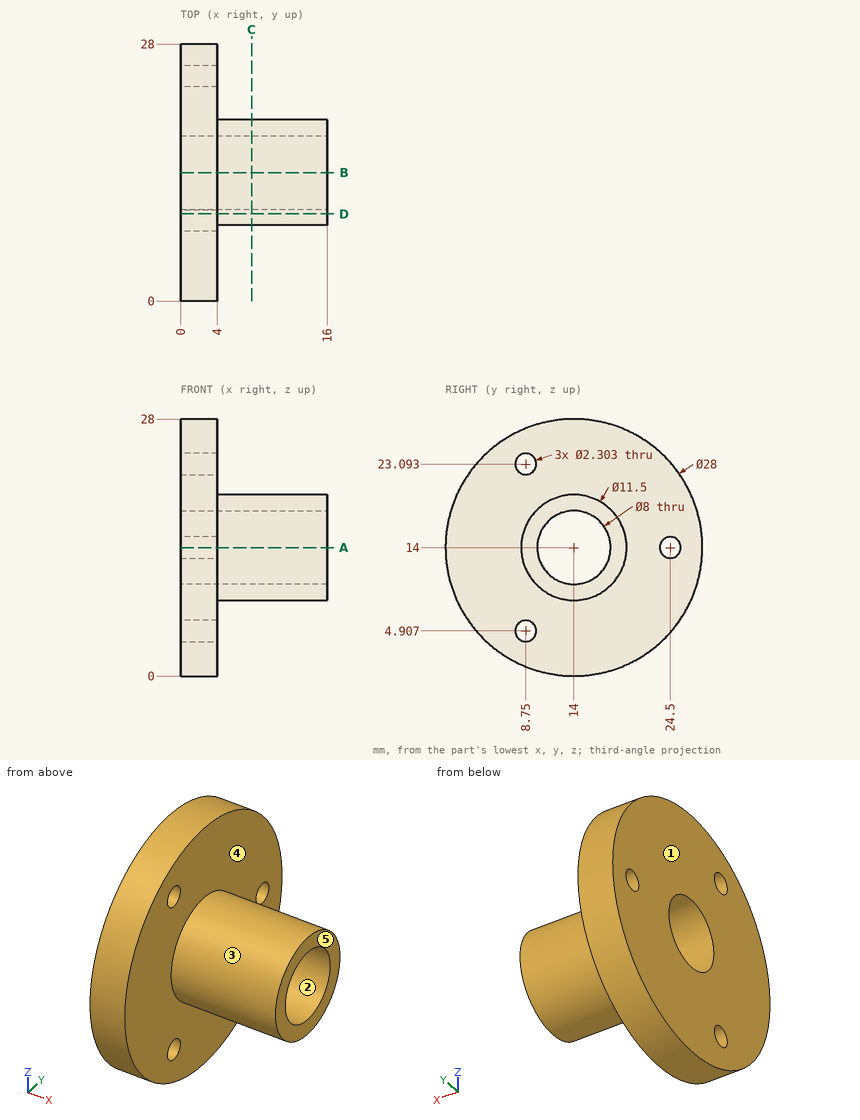
Geometry: see drawing. Coordinates: mm, zero at the bounding-box minimum. A direction names the side the tool comes from. Give positions to 0.01 mm unless a question says otherwise; leave off trailing zeros. Loops run counter-clockwise (first coordinate to the right, second up) from the corner with the lowest first, then second, coordinate; pieces in that order, holes last. Notation, with made-up numbers: (-26, 43.5) - (-1, 43.5) arc R20 ccw to (-1, 55.5) - close; hole circle Ø1 at (-39, 40.25). An arc over 180 degrees is marked (long way). Use CSV: the item, a comma, the result in double quotes. Start each with the question number.
1. Pin query (flat end, axial travel): pin 1 (1 mm diameter, centred on x = 2, y = 16, fed in from -Z); pin 2 (8 mm diameter, centred on y = 18.5, z = 24, fed in from +X); pin 3 (5 mm diameter, centred on x = 13.5, y = 8.5, fed in from -Z) (1 decimal). Return the tip coordinate at first contact, or that it passes through.
2. Section A-A (z = 14). Output: boundary loops of the cut face in (x, y).
3. Reachability of the marked faces 4 and 5 from +Z, -Z, +X, -X, +Y, -Y: full face, straight path, thin tool, end or side. Return the list, or none.
4. Draft query along Y for the marked faces 1, 2 and 3. Return one class per face: +Y half, -Y half, draft (parallel to the pull), parting line (faces both ways), or undercut.
5. Ray query, L1, parallel to Y at x = 1.85, z = 14; L2, parallel to Y at x = 7, z = 14; L3, parallel to X at y = 10.75, z = 1.5. Return the intervals inside material, ascending.
6. Section B-B (y = 14). Output: boundary loops of the cut face in (x, z).
7. Section C-C (x = 7.75). Output: boundary loops of the cut face in (y, z), then the cut area to 3 significant figures.
8. Section D-D (y = 9.5). Output: boundary loops of the cut face in (x, z).
Response:
1,pin 1,"z = 0.08"
1,pin 2,"x = 4"
1,pin 3,"z = 9.1"
2,outline,"(0, 0) - (4, 0) - (4, 8.25) - (16, 8.25) - (16, 10) - (0, 10) - close; (0, 18) - (16, 18) - (16, 19.75) - (4, 19.75) - (4, 23.35) - (0, 23.35) - close; (0, 25.65) - (4, 25.65) - (4, 28) - (0, 28) - close"
3,face 4,"+X"
3,face 5,"+Z, -Z, +X, +Y, -Y"
4,face 1,"draft"
4,face 2,"undercut"
4,face 3,"parting line"
5,L1,"0 to 10, 18 to 23.35, 25.65 to 28"
5,L2,"8.25 to 10, 18 to 19.75"
5,L3,"0 to 4"
6,outline,"(0, 0) - (4, 0) - (4, 8.25) - (16, 8.25) - (16, 10) - (0, 10) - close; (0, 18) - (16, 18) - (16, 19.75) - (4, 19.75) - (4, 28) - (0, 28) - close"
7,outline,"circle Ø11.5 at (14, 14); hole circle Ø8 at (14, 14)"
7,area,"53.6 mm²"
8,outline,"(0, 0.74) - (4, 0.74) - (4, 4.03) - (0, 4.03) - close; (0, 5.78) - (4, 5.78) - (4, 10.42) - (16, 10.42) - (16, 17.58) - (4, 17.58) - (4, 22.22) - (0, 22.22) - close; (0, 23.97) - (4, 23.97) - (4, 27.26) - (0, 27.26) - close"
